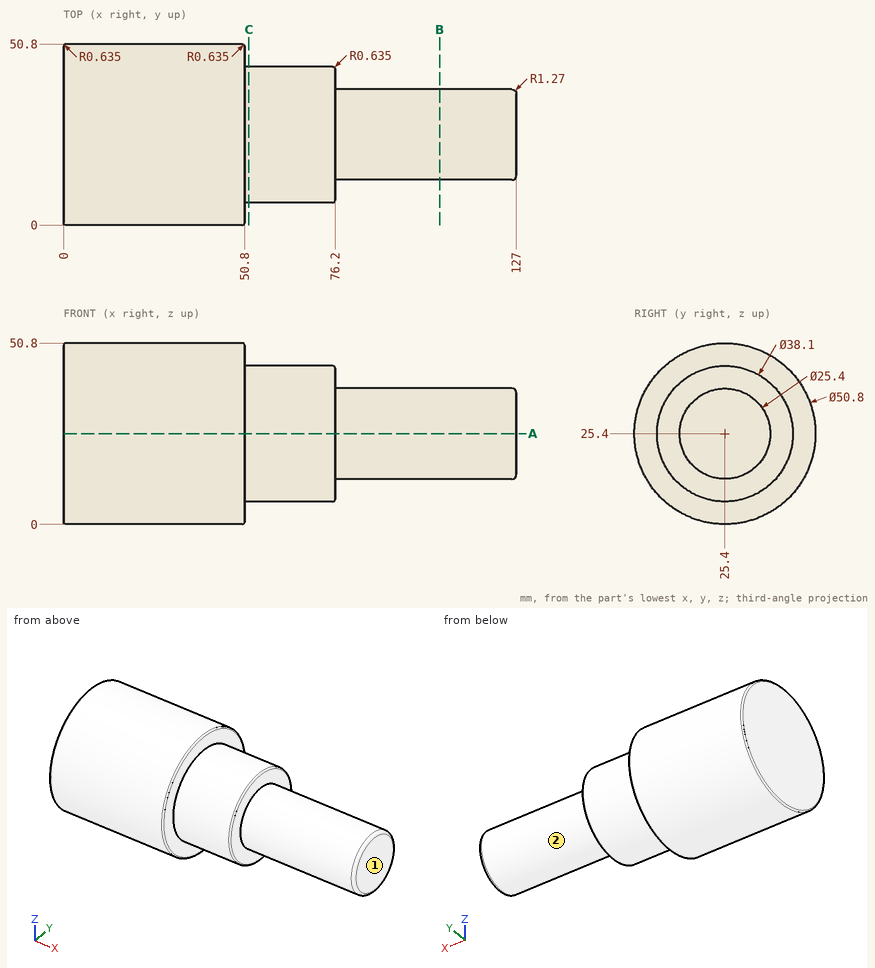
Answer from the drawing. Dimensions are ordinates in mm from the lowest x, y and z of the part. A direction names the side the tool comes from. Round coordinates to 2 decimals unless told otherwise and drop trailing zeros. Order: outer loops, then holes, each group sorted by start corner. A loop starts at its lowest first (then second) coordinate and runs counter-clockwise, first axis right, second up. Notation, with made-up numbers: (67, 34.5) -> (115, 34.5) arc R16 cw to (115, 61.5) -> close; hole circle Ø4 at (33.25, -1.75). An arc over 180 degrees is marked (long way). Answer as CSV lines item,"result".
Q1. Consider line 1 (X direction, y = 39.5, z = 37); line 2 (X direction, y = 16.5, z = 45.5); line 3 (Y direction, x = 95, z = 28). Determine where each line is inside the solid, lowest interval first. Write a range as from..to.
Computed values:
line 1,"x = 0..76.2"
line 2,"x = 0..50.8"
line 3,"y = 12.97..37.83"
Q2. A cutting plane is placed at C-C on x = 52. Determine the outline of the cut face in (y, z).
Computed values:
outline,"circle Ø38.1 at (25.4, 25.4)"
Q3. A cutting plane is placed at B-B on x = 105.5. Determine the outline of the cut face in (y, z), plus the area to 3 significant figures.
Computed values:
outline,"circle Ø25.4 at (25.4, 25.4)"
area,"507 mm^2"
Q4. Which of the six approach directions +Z, -Z, +X, -X, +Y, -Y give full straight-line access (tool end or side, diameter ignored) to the marked faces 1 and 2?
Computed values:
face 1,"+Z, -Z, +X, +Y, -Y"
face 2,"+X"
Q5. Given pin 1 (2 mm diameter, centred on x = 99.5, z = 33, fed in from +Y); pin 2 (2 mm diameter, centred on y = 34.5, z = 38, fed in from +X); pin 3 (3 mm diameter, centred on x = 33.5, z = 10, fed in from +Y), each flat-ended and moving along its own axis, determine where each tip first touches the part or whether it passes through.
Computed values:
pin 1,"stops at y = 36.25"
pin 2,"stops at x = 76.2"
pin 3,"stops at y = 46.66"
Q6. A cutting plane is placed at A-A on z = 25.4. Determine the outline of the cut face in (x, y) (3 decimals).
Computed values:
outline,"(0, 0.635) arc R0.635 ccw to (0.635, 0) -> (50.165, 0) arc R0.635 ccw to (50.8, 0.635) -> (50.8, 6.35) -> (75.565, 6.35) arc R0.635 ccw to (76.2, 6.985) -> (76.2, 12.7) -> (125.73, 12.7) arc R1.27 ccw to (127, 13.97) -> (127, 36.83) arc R1.27 ccw to (125.73, 38.1) -> (76.2, 38.1) -> (76.2, 43.815) arc R0.635 ccw to (75.565, 44.45) -> (50.8, 44.45) -> (50.8, 50.165) arc R0.635 ccw to (50.165, 50.8) -> (0.635, 50.8) arc R0.635 ccw to (0, 50.165) -> close"
